Check sheet for the modelled part. Datum: model origin and axes. Units: mm. Face numbers are marked on the shaded views. A direction names the side the tool comes from. Round coordinates to 2 decimals unless told otherwise and drop trailing zeros. Loops run counter-clockwise (first coordinate to the right, second up) from the corner with the lowest first, then second, coordinate; pieces in that order, holes last. Notation, with made-up numbers: M 40,-8 L 59,-8 A33 cw 59,21 Z; hole C 62.25,12.5 d4. An arc over 180 degrees is marked long. Write item = value, one per line. Start each with the question number.
(1) Cross-section at A-A on y = 96. Record the boundary of the cut face in (x, z).
(2) Cross-section at D-D on x = -27. Record the boundary of the cut face in (y, z), plus the area to 3 significant figures.
(3) Cross-section at B-B on x = 0. Record the boundary of the cut face in (y, z), plus the area to 3 significant figures.
(4) Mould release check, pull along X, two halves, no side actions. Record for the marked faces 3, 4, 5 and 6: pulls with the +X half, pulls with the -X half, needs draft (parallel to the pull), parting line crosses it, or undercut.
(5) Set-up check for the marked faces 1 and 2: record each of +Z, -Z, +X, -X, +Y, -Y from which the full face is reachable in a straight line by a thin tool's end or side.
(6) Cross-section at C-C on z = 0. Record the boundary of the cut face in (x, y).
(7) Go/stop test with flat-tipped pins: P1, Ø12, axis at x = -14.5, y = 101, coming from the +Z side; P2, Ø9.5, axis at y = 134, z = 55.5, coming from the -X side; P3, Ø1.1, axis at x = -104.5, y = 0.5, coming from the -Z side. Record where each tip stops, or that it passes through.
(8) Scan lines: L1, parallel to Z at x = 0, y = 38.5; L2, parallel to Z at x = 0, y = 38; L3, parallel to X at y = 51.5, z = 0. Record each from-to range of solid material in increasing order. Write a range as from..to.
from build123d import *

# Parameters (mm, degrees)
SKETCH2_R           = 55
BOSS_EXTRUDE1_DEPTH = 70
SHELL1_T            = -5
SKETCH4_R           = 125
BOSS_EXTRUDE2_DEPTH = 1
RIB7_REACH          = 192.132
SKETCH3_WALL_W      = 472.644862012
SKETCH3_WALL_H      = 10
CIRPATTERN1_COUNT   = 4
CUT_EXTRUDE1_DEPTH  = 1
CIRPATTERN2_COUNT   = 4
CUT_EXTRUDE2_DEPTH  = 194.455421222
CIRPATTERN3_COUNT   = 4
SKETCH10_W          = 64.387061578
SKETCH10_H          = 55
CUT_EXTRUDE3_DEPTH  = 191.131533418
CIRPATTERN4_COUNT   = 2
CIRPATTERN4_ANGLE   = 90
BOSS_EXTRUDE3_START = -70
SKETCH11_W          = 8.729109108
SKETCH11_H          = 17.418342354
BOSS_EXTRUDE3_DEPTH = 220
CIRPATTERN5_COUNT   = 4


with BuildPart() as part:
    # Sketch2 → Boss-Extrude1 (new body)
    with BuildSketch(Plane(origin=(0, 0, 0), x_dir=(1, 0, 0), z_dir=(0, 1, 0))):
        with Locations(Location((0, 0, 0), (0, 0, 270))):
            Circle(SKETCH2_R)
    extrude(amount=BOSS_EXTRUDE1_DEPTH)

    # Shell1
    shell1_openings = [part.faces().sort_by_distance(p)[0] for p in [
        (0, 70, 0),
    ]]
    offset(amount=SHELL1_T, openings=shell1_openings, kind=Kind.INTERSECTION)

    # Sketch4 → Boss-Extrude2 (add)
    with BuildSketch(Plane(origin=(0, 0, 0), x_dir=(1, 0, 0), z_dir=(0, 1, 0))):
        with Locations(Location((0, 0, 0), (0, 0, 270))):
            Circle(SKETCH4_R)
    extrude(amount=BOSS_EXTRUDE2_DEPTH)

    # Sketch3 wall → Rib7 (add, up to next)
    with BuildSketch(Plane(origin=(87, 32.90951621, 0), x_dir=(0.708107200971, -0.706104943994, 0), z_dir=(0.706104943994, 0.708107200971, 0)), mode=Mode.PRIVATE) as rib7_sk1:
        Rectangle(SKETCH3_WALL_W, SKETCH3_WALL_H)
    rib7_tool1 = extrude(rib7_sk1.sketch, amount=-RIB7_REACH, mode=Mode.PRIVATE) - part.part
    rib7 = rib7_tool1.solids().sort_by_distance((87, 32.90951621, 0))[0]
    add(rib7)

    # CirPattern1: Rib7 ×4 about axis
    cirpattern1_axis = Axis((0, 0, 0), (0, 1, 0))
    for i in range(1, CIRPATTERN1_COUNT):
        add(rib7.rotate(cirpattern1_axis, i * 360 / CIRPATTERN1_COUNT))

    # Sketch5 → Cut-Extrude1 (cut)
    with BuildSketch(Plane(origin=(0, 1, 0), x_dir=(1, 0, 0), z_dir=(0, 1, 0))):
        with BuildLine():
            Line((9.493142678, -59.24424227), (9.493142678, -129.652922227))
            ThreePointArc((9.493142678, -129.652922227), (92.201319164, -91.645604065), (129.707942461, -8.709171177))
            Line((129.707942461, -8.709171177), (59.364554554, -8.709171177))
            ThreePointArc((59.364554554, -8.709171177), (42.705900876, -42.145059383), (9.493142678, -59.24424227))
        make_face()
    cut_extrude1 = extrude(amount=-CUT_EXTRUDE1_DEPTH, mode=Mode.SUBTRACT)

    # CirPattern2: Cut-Extrude1 ×4 about axis
    cirpattern2_axis = Axis((0, 0, 0), (0, 1, 0))
    for i in range(1, CIRPATTERN2_COUNT):
        add(cut_extrude1.rotate(cirpattern2_axis, i * 360 / CIRPATTERN2_COUNT), mode=Mode.SUBTRACT)

    # Sketch7 → Cut-Extrude2 (cut, through all)
    with BuildSketch(Plane(origin=(5, 0, 0), x_dir=(0, 0, -1), z_dir=(1, 0, 0))):
        Polygon((59.772255751, 52.99919304), (106.904721419, 6), (59.772255751, 6), align=None)
    cut_extrude2 = extrude(amount=-CUT_EXTRUDE2_DEPTH, mode=Mode.SUBTRACT)

    # CirPattern3: Cut-Extrude2 ×4 about axis
    cirpattern3_axis = Axis((0, 0, 0), (0, 1, 0))
    for i in range(1, CIRPATTERN3_COUNT):
        add(cut_extrude2.rotate(cirpattern3_axis, i * 360 / CIRPATTERN3_COUNT), mode=Mode.SUBTRACT)

    # Sketch10 → Cut-Extrude3 (cut, symmetric)
    with BuildSketch(Plane(origin=(0, 0, 0), x_dir=(0.7117650145966598, -3.2873850610052313e-15, 0.7024176563813135), z_dir=(-0.7024176563813135, -3.331131634682351e-15, 0.7117650145966598))):
        with Locations((-0.279356343, 36.5)):
            Rectangle(SKETCH10_W, SKETCH10_H)
    cut_extrude3 = extrude(amount=CUT_EXTRUDE3_DEPTH, both=True, mode=Mode.SUBTRACT)

    # CirPattern4: Cut-Extrude3 ×2 about axis
    cirpattern4_axis = Axis((0, 70, 0), (0, 1, 0))
    for i in range(1, CIRPATTERN4_COUNT):
        add(cut_extrude3.rotate(cirpattern4_axis, i * CIRPATTERN4_ANGLE / (CIRPATTERN4_COUNT - 1)), mode=Mode.SUBTRACT)

    # Sketch11 → Boss-Extrude3 (add)
    with BuildSketch(Plane(origin=(0, 70, 0), x_dir=(1, 0, 0), z_dir=(0, 1, 0)).offset(BOSS_EXTRUDE3_START)):
        with Locations((55, 0)):
            Rectangle(SKETCH11_W, SKETCH11_H)
    boss_extrude3 = extrude(amount=BOSS_EXTRUDE3_DEPTH)

    # CirPattern5: Boss-Extrude3 ×4 about axis
    cirpattern5_axis = Axis((0, 0, 0), (0, 1, 0))
    for i in range(1, CIRPATTERN5_COUNT):
        add(boss_extrude3.rotate(cirpattern5_axis, i * 360 / CIRPATTERN5_COUNT))


solid = part.part
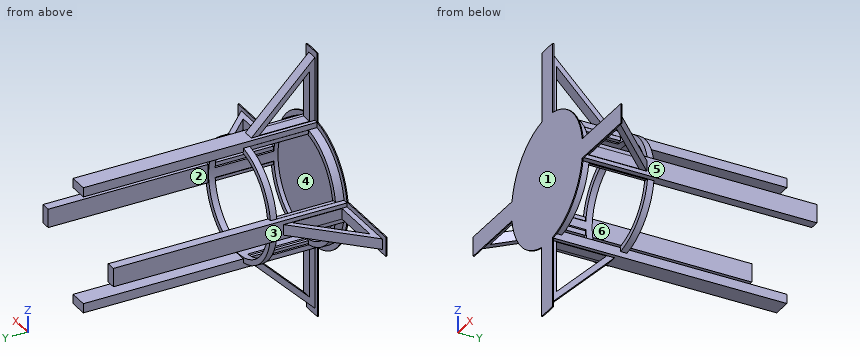
Result:
q1.outline = M -59.36,-8.71 L -50.64,-8.71 L -50.64,8.71 L -59.36,8.71 Z; M -8.71,-59.36 L 8.71,-59.36 L 8.71,-50.64 L -8.71,-50.64 Z; M -8.71,50.64 L 8.71,50.64 L 8.71,59.36 L -8.71,59.36 Z; M 50.64,-8.71 L 59.36,-8.71 L 59.36,8.71 L 50.64,8.71 Z
q2.outline = M 0,-53.58 L 1,-53.58 L 1,-47.92 L 9,-47.92 L 9,-42.08 L 5,-42.08 L 5,42.08 L 9,42.08 L 9,47.92 L 1,47.92 L 1,53.58 L 0,53.58 Z; M 64,-47.92 L 70,-47.92 L 70,-42.08 L 64,-42.08 Z; M 64,42.08 L 70,42.08 L 70,47.92 L 64,47.92 Z
q2.area = 607 mm^2
q3.outline = M 0,-125 L 1,-125 L 1,-119 L 60.47,-59.36 L 220,-59.36 L 220,-50.64 L 70,-50.64 L 70,-50 L 5,-50 L 5,50 L 70,50 L 70,50.64 L 220,50.64 L 220,59.36 L 60.47,59.36 L 1,119 L 1,125 L 0,125 Z; hole M 6,-106.9 L 53,-59.77 L 6,-59.77 Z; hole M 6,59.77 L 53,59.77 L 6,106.9 Z
q3.area = 5,890 mm^2
q4.face_3 = pulls with the -X half
q4.face_4 = undercut
q4.face_5 = pulls with the +X half
q4.face_6 = undercut
q5.face_1 = +Z, -Z, +X, -X, -Y
q5.face_2 = +Z, -Z, +Y
q6.outline = M -125,0 L 125,0 L 125,1 L 119,1 L 59.36,60.47 L 59.36,220 L 50.64,220 L 50.64,70 L 50,70 L 50,5 L -50,5 L -50,70 L -50.64,70 L -50.64,220 L -59.36,220 L -59.36,60.47 L -119,1 L -125,1 Z; hole M -106.9,6 L -59.77,6 L -59.77,53 Z; hole M 59.77,6 L 106.9,6 L 59.77,53 Z
q7.P1 = 59.36
q7.P2 = -8.71
q7.P3 = -8.71
q8.L1 = -81.39..-74.31, -59.77..-50, 50..59.77, 74.31..81.39
q8.L2 = -81.9..-74.81, -59.77..-50, 50..59.77, 74.81..81.9
q8.L3 = -68.36..-61.28, -59.77..-50, 50..59.77, 61.28..68.36
